Can you work these out from the drawing? Everything is in mm from the part's minimum corner. A direction names the side the tool comes from. Round coordinates to 2 decimals unless told otherwise and drop trailing zeros. Write each loop counter-clockwise with the first axis right and the second up, starting at its lowest first coordinate (ties: lowest second). Pieces come first, ordered by that corner, then holes. Notation, with made-up numbers: (88.25, 50.5) - (113.25, 50.5) arc R13 ccw to (113.25, 66.5) - close; hole circle Ø9 at (39, -33). An arc over 180 degrees is marked (long way). Write each question's results on one line, items separated by ' | '. Start each with the question number.
(1) Imagine slicing it at D-D on y = 8. Write out the boundary of the cut face in (x, z) (3 decimals).
(2) Imagine slicing it at B-B on z = 12. Write out the boundary of the cut face in (x, y).
(3) Thinking about a two-plate mould opening in X: for the marked faces 3, 4 and 5, which applies, +X half, -X half, draft (parallel to the pull), parting line (faces both ways), or undercut?
(4) Please list where these lines run through material, in increasing order: line 1 (Z direction, x = 84, y = 52) (3 decimals); line 2 (X direction, y = 51.35, z = 5); line 3 (X direction, y = 51, z = 5). Write a range as [from, to].
(5) Imagine slicing it at A-A on y = 18. Write out the boundary of the cut face in (x, z) (3 decimals).
(6) Imagine slicing it at C-C on x = 120. Write out the boundary of the cut face in (y, z) (3 decimals), then the cut area to 3 significant figures.
(7) For P1, Ø4, axis at y = 9, z = 6.5, coming from the -X side; P2, Ø6, axis at x = 146.75, z = 5, coming from the -Y side; P3, Ø1, axis at y = 22, z = 32, coming from the +X side; P4, Ø3, axis at x = 84.25, z = 5, coming from the +Y side, each with a flat end and sliding along its axis, tell me the tip position at first contact or that it passes through.
(8) On a 3-axis mill with a long thin cutter (end or side, diameter ignored), from which of +Z, -Z, +X, -X, +Y, -Y can I reach the whole of each face in a straight line? I mean the marked faces 1 and 2. Say none if no direction works.
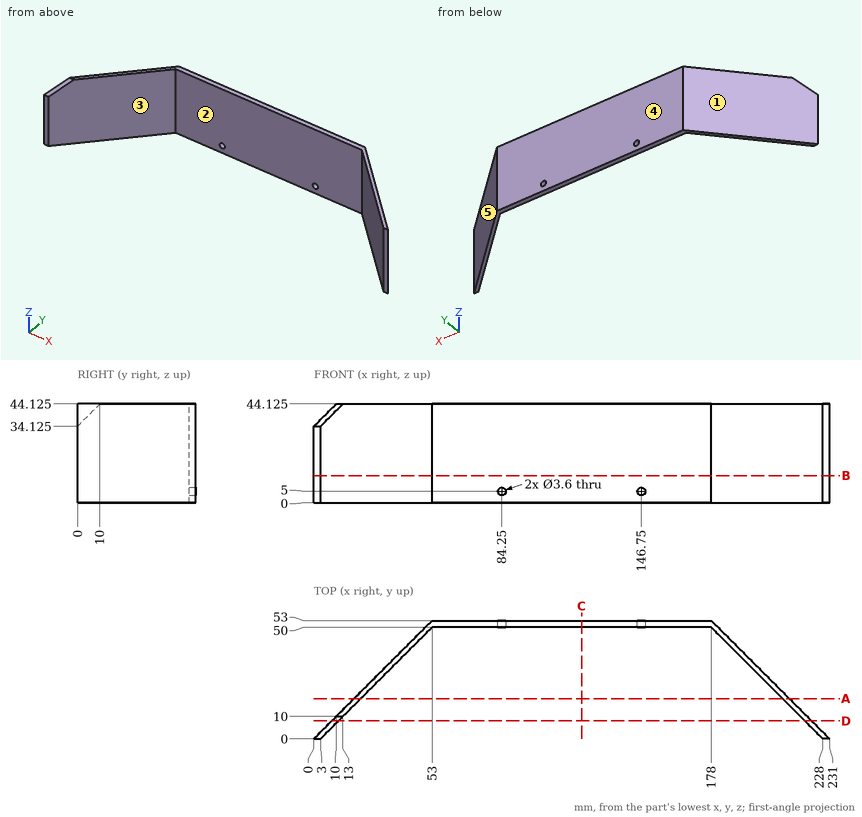
Response:
1) outline: (8, 0) - (11, 0) - (11, 42.125) - (8, 42.125) - close; (220, 0) - (223, 0) - (223, 44.125) - (220, 44.125) - close
2) outline: (0, 0) - (3, 0) - (53, 50) - (178, 50) - (228, 0) - (231, 0) - (178, 53) - (53, 53) - close
3) face 3: undercut | face 4: draft | face 5: +X half
4) line 1: [0, 3.217], [6.783, 44.125] | line 2: [51.35, 82.45], [86.05, 144.95], [148.55, 179.65] | line 3: [51, 82.45], [86.05, 144.95], [148.55, 180]
5) outline: (18, 0) - (21, 0) - (21, 44.125) - (18, 44.125) - close; (210, 0) - (213, 0) - (213, 44.125) - (210, 44.125) - close
6) outline: (50, 0) - (53, 0) - (53, 44.125) - (50, 44.125) - close | area: 132 mm²
7) P1: x = 7 | P2: y = 50 | P3: x = 209.5 | P4: through
8) face 1: +Z, -Z, -X, +Y | face 2: +Z, -Z, -Y
